Study the drawing (mm; zero at the part's minimum x, y, z) and answer. Coordinates: 2 decimals unless noted, no trailing zeros. Write each loop counter-clockwise with the first axis right and the second up, starting at its lowest first coordinate (ties: lowest second). Pieces come first, ordered by that corner, then holes. Notation, with made-up numbers: (52, 6.5) - (99, 6.5) arc R26 ccw to (99, 45.5) - close; hole circle Ø4 at (5, 5.5). An arc over 180 degrees is marked (long way). One line per item, written item: value.
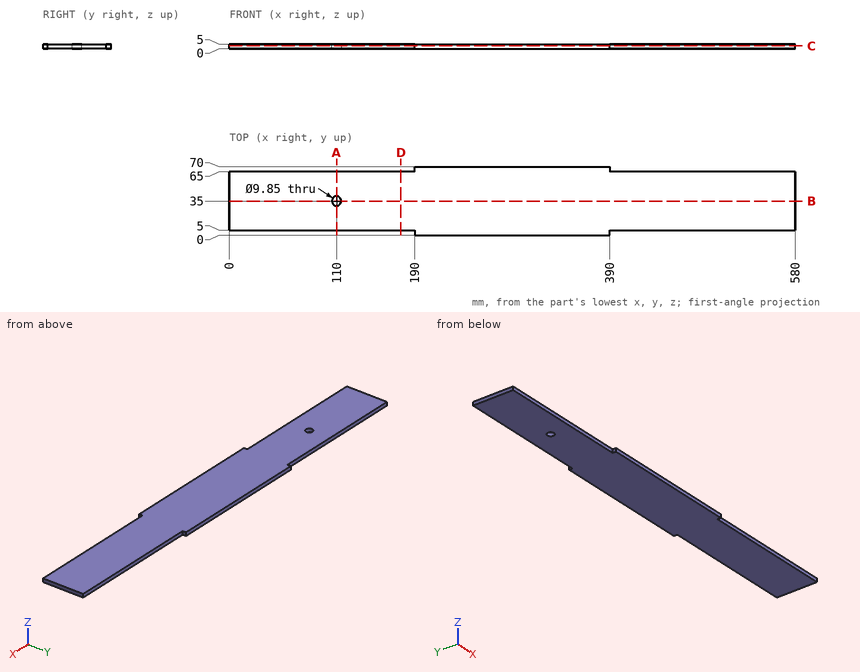
Item 1: Given pin 1 (2.5 mm diameter, centred on y = 1.5, z = 1.5, fed in from +X); pin 2 (2.5 mm diameter, centred on x = 522.5, z = 1.5, fed in from +Y); pin 3 (2.5 mm diameter, centred on y = 3, z = 3, fed in from -X), each flat-ended and moving along its own axis, determine where each tip first touches the part or whether it passes through.
Evaluation:
pin 1: stops at x = 390
pin 2: stops at y = 65
pin 3: stops at x = 190
Item 2: Consider probe 1 along Y at (x, z) = (110, 3.15) (3 decimals); probe 2 along Y at (x, z) = (436.5, 4). Determine where each line is inside the solid, lowest interval first.
Evaluation:
probe 1: y = 5 to 30.075, 39.925 to 65
probe 2: y = 5 to 65
Item 3: Section D-D, the plane x = 176 is taken. Determine the outline of the cut face in (y, z).
Evaluation:
outline: (5, 0) - (65, 0) - (65, 5) - (5, 5) - close
Item 4: Section A-A, the plane x = 110 is taken. Determine the outline of the cut face in (y, z) (3 decimals).
Evaluation:
outline: (5, 0) - (30.075, 0) - (30.075, 5) - (5, 5) - close; (39.925, 0) - (65, 0) - (65, 5) - (39.925, 5) - close
Item 5: Section C-C, the plane z = 3.15 is taken. Determine the outline of the cut face in (x, y) (3 decimals), then the cut area to 3 significant figures.
Evaluation:
outline: (0, 5) - (190, 5) - (190, 0) - (390, 0) - (390, 5) - (580, 5) - (580, 65) - (390, 65) - (390, 70) - (190, 70) - (190, 65) - (0, 65) - close; hole circle Ø9.85 at (110, 35)
area: 36,700 mm2
Item 6: Section B-B, the plane y = 35 is taken. Determine the outline of the cut face in (x, z) (3 decimals).
Evaluation:
outline: (0, 0) - (105.075, 0) - (105.075, 5) - (0, 5) - close; (114.925, 0) - (580, 0) - (580, 5) - (114.925, 5) - close
